from build123d import *

# Parameters (mm, degrees)
BOSS_EXTRUDE1_DEPTH = 2.54
SKETCH2_R           = 25.4
BOSS_EXTRUDE2_DEPTH = 1828.8
BOSS_EXTRUDE3_DEPTH = 2.54
SKETCH4_R           = 31.109831221
BOSS_EXTRUDE5_DEPTH = 76.2
SKETCH5_W           = 36.901431936
SKETCH5_H           = 931.81733007
BOSS_EXTRUDE7_DEPTH = 50.8
BOSS_EXTRUDE8_DEPTH = 38.1


with BuildPart() as part:
    # Sketch1 → Boss-Extrude1 (new body)
    with BuildSketch(Plane(origin=(0, 0, 0), x_dir=(1, 0, 0), z_dir=(0, 1, 0))):
        Polygon((0, -304.8), (263.964543074, 152.4), (-263.964543074, 152.4), align=None)
    extrude(amount=BOSS_EXTRUDE1_DEPTH)

    # Sketch2 → Boss-Extrude2 (add)
    with BuildSketch(Plane(origin=(0, 2.54, 0), x_dir=(1, 0, 0), z_dir=(0, 1, 0))):
        with Locations(Location((0, -304.8, 0), (0, 0, 120))):
            Circle(SKETCH2_R)
        with Locations((-263.964543074, 152.4)):
            Circle(SKETCH2_R)
        with Locations(Location((263.964543074, 152.4, 0), (0, 0, 180))):
            Circle(SKETCH2_R)
    extrude(amount=BOSS_EXTRUDE2_DEPTH)

    # Sketch3 → Boss-Extrude3 (add)
    with BuildSketch(Plane(origin=(0, 1831.34, 0), x_dir=(1, 0, 0), z_dir=(0, 1, 0))):
        Polygon((-263.964543074, 152.4), (0, -307.726008903), (265.059219048, 152.4), align=None)
    extrude(amount=BOSS_EXTRUDE3_DEPTH)

    # Sketch4 → Boss-Extrude5 (add)
    with BuildSketch(Plane(origin=(0, 1833.88, 0), x_dir=(1, 0, 0), z_dir=(0, 1, 0))):
        with Locations(Location((0, 0, 0), (0, 0, 90))):
            Circle(SKETCH4_R)
    extrude(amount=BOSS_EXTRUDE5_DEPTH)

    # Sketch5 → Boss-Extrude7 (add)
    with BuildSketch(Plane(origin=(0, 1910.08, 0), x_dir=(1, 0, 0), z_dir=(0, 1, 0))):
        Rectangle(SKETCH5_W, SKETCH5_H)
    extrude(amount=BOSS_EXTRUDE7_DEPTH)

    # 3DSketch1 → Boss-Extrude8 (add)
    with BuildSketch(Plane(origin=(327.254814747, 1315.114471395, -152.4), x_dir=(-0.8541064020391608, -0.5200983118562486, 0), z_dir=(0, 0, 1))):
        Polygon((0, 0), (554.560573308, -337.693310003), (760.195046997, 0), (205.634473689, 337.693310003), align=None)
    extrude(amount=-BOSS_EXTRUDE8_DEPTH)


solid = part.part
CAD build for the part. Positions are in the model's coordinates, mm. A direction names the side the tool comes from. Give positions to 0.01 mm unless a question says otherwise; leave off trailing zeros. Write each loop counter-clockwise with the first axis right and the second up, starting at its lowest first coordinate (ties: lowest second). Pieces come first, ordered by that corner, then holes. Notation, with made-up numbers: (-26.75, 73.25) - (15.25, 73.25) arc R20 ccw to (15.25, 111.25) - close; hole circle Ø8 at (0, -16). An arc over 180 degrees is marked (long way). Put each result on its own line as item: value.
(1) Pull direction X, two halves, no side cores. Call faces 6 (the flat face through (6, 1116, -152.4)), 7 (the flat face through (-4, 0, 22)), 8 (the flat face through (327.255, 1115, -171)): released by +X, released by -X, zero draft, split by the parting line, or undercut.
Working result:
face 6: undercut
face 7: zero draft
face 8: released by +X
(2) Wall check: L1, parallel to Y at x = -126.5, z = -13; L2, parallel to Y at x = -16, z = -263.5; L3, parallel to Y at x = -198.5, z = -174.5. Give the ranges that are in metal, low to high.
Working result:
L1: 0 to 2.54, 1831.34 to 1833.88
L2: 1910.08 to 1960.88
L3: 919.74 to 1315.11
(3) Saw through at A-A (x = 107). List the corners of the cut face in (y, z).
Working result:
outline: (0, -152.4) - (2.54, -152.4) - (2.54, 119.47) - (0, 119.47) - close; (919.74, -190.5) - (1315.11, -190.5) - (1315.11, -152.4) - (919.74, -152.4) - close; (1831.34, -152.4) - (1833.88, -152.4) - (1833.88, 121.98) - (1831.34, 121.98) - close
(4) Drop flat-ended pins along their axis: pin 1 Ø6 at (y, z) = (1133.5, 326) entering from +X; pin 2 Ø18.5 at (x, z) = (-8, -177) entering from -Y; pin 3 Ø5 at (x, y) = (243, 806) entering from -Z; pin 4 Ø8 at (x, z) = (174, -136) entering from -Y. Give the stop position or say it passes through.
Working result:
pin 1: x = 17.72
pin 2: y = 919.74
pin 3: z = -169.84
pin 4: y = 0
(5) Tool access for faces 1 (the flat face through (309, 1117, -152.4)), 2 (the flat face through (3, 1831.34, 310)), 3 (the flat face through (-322.033, 1120, -171)), 4 (the flat face through (130.135, 1.252, 79.4)), 5 (the cylindrical face through (267.271, 904.138, -127.216)): list every direction of +Z, -Z, +X, -X, +Y, -Y with a clear straight run to the whole face (end or side of a thin tool).
Working result:
face 1: +Z, +X, +Y, -Y
face 2: +Z
face 3: +Z, -Z, -X, +Y, -Y
face 4: +Z, +X, -Y
face 5: none
(6) Saw through at C-C (z = 0). List the corners of the cut face in (x, y).
Working result:
outline: (-176.54, 1831.34) - (177.27, 1831.34) - (177.27, 1833.88) - (31.11, 1833.88) - (31.11, 1910.08) - (18.45, 1910.08) - (18.45, 1960.88) - (-18.45, 1960.88) - (-18.45, 1910.08) - (-31.11, 1910.08) - (-31.11, 1833.88) - (-176.54, 1833.88) - close; (-175.98, 0) - (175.98, 0) - (175.98, 2.54) - (-175.98, 2.54) - close
(7) Saw through at D-D (x = -157.5). List the corners of the cut face in (y, z).
Working result:
outline: (0, -152.4) - (2.54, -152.4) - (2.54, 32) - (0, 32) - close; (919.74, -190.5) - (1315.11, -190.5) - (1315.11, -152.4) - (919.74, -152.4) - close; (1831.34, -152.4) - (1833.88, -152.4) - (1833.88, 33.18) - (1831.34, 33.18) - close
(8) Saw through at B-B (y = 287.5). List the corners of the cut face in (x, z).
Working result:
outline: circle Ø50.8 at (-263.96, -152.4); circle Ø50.8 at (0, 304.8); circle Ø50.8 at (263.96, -152.4)
